Verification items for the finished model (mm, model axes). A direction names the side the tool comes from. Coordinates: 2 decimals unless noted, no trailing zeros. Write each loop counter-clockwise with the first axis right and the second up, starting at its lowest first coordinate (ties: lowest second). Pieces come first, ordered by that corner, then holes. Notation, with made-up numbers: (63, 42.25) -> (73, 42.25) arc R16 ccw to (73, 67.25) -> close; hole circle Ø7 at (-35, -8.5). An arc over 180 degrees is marked (long way). Write item = value, one per line. Start each with the question number.
(1) Gauge pin test, flat ends, axial feed: pin 1 Ø8 at (x, z) = (31.16, 6.44) entering from -Y; pin 2 Ø10 at (y, z) = (17, 6) entering from +X; pin 3 Ø4 at (x, y) = (6, 24) entering from -Z. Record the tip position at first contact, or that the pin passes through.
(2) Section check C-C (z = 2.75). Record the cut outline in (x, y), plus the area to 3 significant figures.
(3) Set-up check for faces 4 (the face through (42.135, 14.951, 12.522)), 5 (the face through (5, 0, 25.4)), 6 (the face through (10, -19.398, 6)), 7 (the face through (-16.18, -4.21, 22.27)), 8 (the face through (3, 22, 12.7)): record each of +Z, -Z, +X, -X, +Y, -Y from which the full face is reachable in a straight line by a thin tool's end or side.
(4) Material ranges on probe 1 along Z at (x, y) = (10, -19.5); probe 2 along X at (y, z) = (-5.5, 5.25); probe 3 along Y at (x, z) = (-17, 20.5), recorded low to high. Write a range as [from, to].
(5) Section check A-A (x = 16). Record the cut outline in (y, z), plus the area to 3 significant figures.
(6) Mould release check, pull along X, two halves, no side actions. Record for faces 1 (the face through (32.29, -2.15, 4.27)), 2 (the face through (0, -28.569, 19)), 3 (the face through (40.58, -1.34, 20.55)): released by +X, released by -X, zero draft, split by the parting line, or undercut.
(7) Section check D-D (x = 29.5). Record the cut outline in (y, z), plus the area to 3 significant figures.
(8) Section check B-B (y = 0). Record the cut outline in (x, z), plus the area to 3 significant figures.
```python
from build123d import *

# Parameters (mm, degrees)
F0_R     = 4.149951
F1_DEPTH = 25.4
F3_DEPTH = 50.8
F5_DEPTH = 12.7
F6_R     = 6.918171
F7_DEPTH = 6.35
F8_R     = 2.452339
F9_DEPTH = 47.968393


with BuildPart() as f1:
    # F0 (on Top) → F1 (new body)
    with BuildSketch(Plane.XY):
        Polygon((20.776082, 28.569183), (-20.776082, 28.569183), (-20.776082, -28.569183), (20.776082, -28.569183), (55.331081, -13.142847), (55.331081, 6.537836), align=None)
        with Locations((-10.68896, 0)):
            Circle(F0_R, mode=Mode.SUBTRACT)
    extrude(amount=F1_DEPTH)

    # F2 (on Front) → F3 (cut, symmetric)
    with BuildSketch(Plane.XZ):
        Polygon((31.462464, 25.4), (55.331081, 12.7), (55.331081, 25.4), align=None)
    extrude(amount=F3_DEPTH, both=True, mode=Mode.SUBTRACT)

    # F4 (on face) → F5 (cut)
    with BuildSketch(Plane(origin=(0, 0, 0), x_dir=(1, 0, 0), z_dir=(0, 0, -1))):
        Polygon((20.776082, 28.569183), (-20.776082, 28.569183), (-20.776082, 19.398211), (41.319063, 19.398211), align=None)
        Polygon((41.120535, -15.598102), (-20.776082, -15.598102), (-20.776082, -28.569183), (20.776082, -28.569183), align=None)
    extrude(amount=-F5_DEPTH, mode=Mode.SUBTRACT)

    # F6 (on face) → F7 (cut)
    with BuildSketch(Plane.XY.offset(25.4)):
        with Locations((-10.68896, 0)):
            Circle(F6_R)
    extrude(amount=-F7_DEPTH, mode=Mode.SUBTRACT)

    # F8 (on face) → F9 (cut, through all)
    with BuildSketch(Plane.XZ.offset(19.398211)):
        with Locations((31.159063, 6.444813)):
            Circle(F8_R)
    extrude(amount=-F9_DEPTH, mode=Mode.SUBTRACT)


solid = f1.part
```
Response:
q1.pin_1 = -19.4
q1.pin_2 = 46.76
q1.pin_3 = 12.7
q2.outline = (-20.78, -19.4) -> (41.32, -19.4) -> (55.33, -13.14) -> (55.33, 6.54) -> (41.12, 15.6) -> (-20.78, 15.6) -> close; hole circle Ø8.3 at (-10.69, 0)
q2.area = 2,500 mm2
q3.face_4 = +Z, -Z, +X, +Y
q3.face_5 = +Z, +X, -X, +Y, -Y
q3.face_6 = -Z, +X, -X, -Y
q3.face_7 = +Z
q3.face_8 = -Z, +X, -X, +Y
q4.probe_1 = [12.7, 25.4]
q4.probe_2 = [-20.78, 29.02], [33.3, 55.33]
q4.probe_3 = [-28.57, -2.83], [2.83, 28.57]
q5.outline = (-28.57, 12.7) -> (-19.4, 12.7) -> (-19.4, 0) -> (15.6, 0) -> (15.6, 12.7) -> (28.57, 12.7) -> (28.57, 25.4) -> (-28.57, 25.4) -> close
q5.area = 1,170 mm2
q6.face_1 = undercut
q6.face_2 = zero draft
q6.face_3 = released by +X
q7.outline = (-24.67, 12.7) -> (-19.4, 12.7) -> (-19.4, 8.25) -> (15.6, 8.25) -> (15.6, 12.7) -> (23.01, 12.7) -> (23.01, 25.4) -> (-24.67, 25.4) -> close; (-19.4, 0) -> (15.6, 0) -> (15.6, 4.64) -> (-19.4, 4.64) -> close
q7.area = 924 mm2
q8.outline = (-20.78, 0) -> (-14.84, 0) -> (-14.84, 19.05) -> (-17.61, 19.05) -> (-17.61, 25.4) -> (-20.78, 25.4) -> close; (-6.54, 0) -> (55.33, 0) -> (55.33, 12.7) -> (31.46, 25.4) -> (-3.77, 25.4) -> (-3.77, 19.05) -> (-6.54, 19.05) -> close; hole circle Ø4.9 at (31.16, 6.44)
q8.area = 1,520 mm2
